Job drawing, mm, ordinate dimensions from the low corner. One solid piece. Round coordinates to 2 decimals unless told otherwise and drop trailing zeros. Loops run counter-clockwise (first coordinate to the right, second up) from the corner with the lowest first, then second, coordinate; pieces in that order, holes last. Notation, with made-up numbers: M -28,50 L -21,50 A23 ccw -21,86 Z; hole C 84,57 d9. An arc over 180 degrees is marked long. Use a Markdown table: item, result. Add a question column.
(1) Wall check: L1, parallel to Y at x = 68.2, z = 1.65; L2, parallel to X at y = 38.1, z = 0.65; L3, parallel to X at y = 67.5, z = 2.65. Give the ranges that are in metal, low to high.
(2) Band-saw the part on A-A, the plane x = 38.1. Write the cut outline in (y, z), and give its area (3 significant figures).
(3) Flat gauge pin, fed straight in: P1, Ø5, axis at x = 58.5, y = 33.5, coming from the +Z side. Where does the tip first touch, or does it go through?
(4) Band-saw the part on C-C, the plane z = 2.5. Write the cut outline in (x, y), and give its area (3 significant figures).
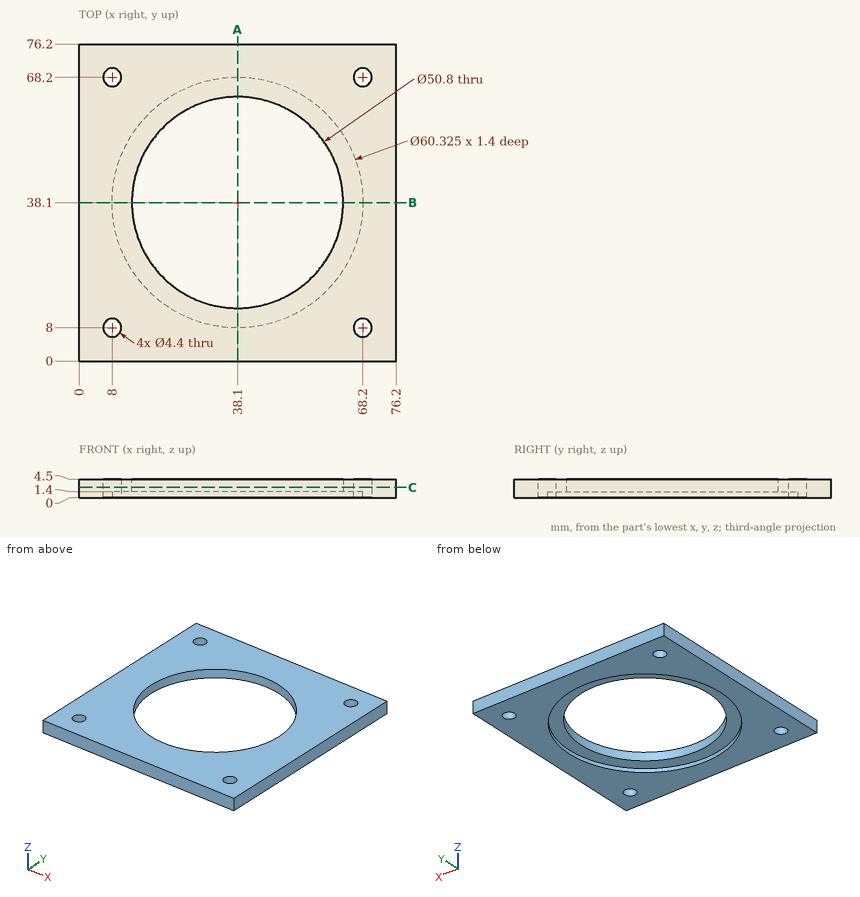
Return value:
| question | item | result |
|---|---|---|
| 1 | L1 | 0 to 5.8, 10.2 to 66, 70.4 to 76.2 |
| 1 | L2 | 0 to 7.94, 68.26 to 76.2 |
| 1 | L3 | 0 to 5.91, 10.09 to 66.11, 70.29 to 76.2 |
| 2 | outline | M 0,0 L 7.94,0 L 7.94,1.4 L 12.7,1.4 L 12.7,4.5 L 0,4.5 Z; M 63.5,1.4 L 68.26,1.4 L 68.26,0 L 76.2,0 L 76.2,4.5 L 63.5,4.5 Z |
| 2 | area | 101 mm^2 |
| 3 | P1 | through |
| 4 | outline | M 0,0 L 76.2,0 L 76.2,76.2 L 0,76.2 Z; hole C 8,8 d4.4; hole C 8,68.2 d4.4; hole C 38.1,38.1 d50.8; hole C 68.2,8 d4.4; hole C 68.2,68.2 d4.4 |
| 4 | area | 3,720 mm^2 |
